Could you check a few things on this model? Use its own coordinates, in mm. Face numbers are marked on the shaded views. A direction names the side the tool comes from. Round coordinates to 2 decimals unless told otherwise and drop trailing zeros. Loops run counter-clockwise (first coordinate to the right, second up) from the corner with the lowest first, then second, coordinate; pieces in that order, holes last. Notation, with made-up numbers: (67.5, -12) - (84.5, -12) arc R21 cw to (84.5, -2) - close; hole circle Ø11 at (59, 28.25). An arc over 180 degrees is marked (long way). Use one line per item in the form item = value.
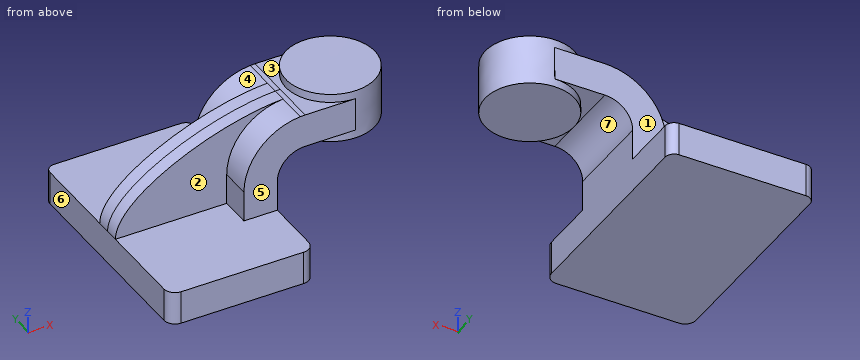
```python
from build123d import *

# Parameters (mm, degrees)
F1_DEPTH = 63.5
F2_DEPTH = 7.9375
F3_DEPTH = 25.4
F5_R     = 6.35
F6_R     = 5.08


with BuildPart() as f1:
    # F0 (on Front) → F1 (new body, symmetric)
    with BuildSketch(Plane.XZ):
        Polygon((-41.275, -9.525), (41.275, -9.525), (41.275, 9.525), (22.225, 9.525), (-41.275, 9.525), align=None)
    extrude(amount=F1_DEPTH, both=True)

    # F0 (on Front) → F2 (join, symmetric)
    with BuildSketch(Plane.XZ):
        with BuildLine():
            add(Edge.make_bspline(
                [(-41.275, 9.525), (-41.1638136776, 33.0921679971), (14.6157059848, 59.6638127103), (54.3682484127, 61.8142414647)],
                knots=[0, 0, 0, 0, 108.9382602659, 108.9382602659, 108.9382602659, 108.9382602659], degree=3))
            Line((-41.275, 9.525), (22.225, 9.525))
            Line((22.225, 9.525), (22.225, 27.0002))
            ThreePointArc((22.225, 27.0002), (31.489638553, 50.6920018607), (54.3682484127, 61.8142414647))
        make_face()
    extrude(amount=F2_DEPTH, both=True)

    # F0 (on Front) → F3 (join, symmetric)
    with BuildSketch(Plane.XZ):
        with BuildLine():
            Line((22.225, 9.525), (41.275, 9.525))
            Line((41.275, 9.525), (41.275, 27.0002))
            ThreePointArc((41.275, 27.0002), (45.9246798487, 38.2255201513), (57.15, 42.8752))
            Line((57.15, 42.8752), (60.325, 42.8752))
            Line((60.325, 42.8752), (60.325, 61.9252))
            Line((60.325, 61.9252), (57.15, 61.9252))
            add(Edge.make_bspline(
                [(54.3682484127, 61.8142414647), (55.3047053678, 61.8648994564), (56.2322683165, 61.902005145), (57.15, 61.9252)],
                knots=[108.9382602659, 108.9382602659, 108.9382602659, 108.9382602659, 111.5045361635, 111.5045361635, 111.5045361635, 111.5045361635], degree=3))
            ThreePointArc((54.3682484127, 61.8142414647), (31.489638553, 50.6920018607), (22.225, 27.0002))
            Line((22.225, 27.0002), (22.225, 9.525))
        make_face()
        Polygon((60.325, 61.9252), (60.325, 42.8752), (85.7332489532, 42.8752), (85.7661570114, 61.9252), align=None)
    extrude(amount=F3_DEPTH, both=True)

    # F0 (on Front) → F4 (revolve)
    with BuildSketch(Plane.XZ):
        Polygon((85.7661570114, 61.9252), (85.7332489532, 42.8752), (85.725, 38.1), (111.125, 38.1), (111.125, 66.675), (85.7743620872, 66.675), align=None)
    revolve(axis=Axis((85.7496810436, 0, 52.3875), (0.0017274545, 0, 0.9999985079)))

    # F5
    f5_edges = [f1.edges().sort_by_distance(p)[0] for p in [
        (41.275, -63.5, 0),
        (-41.275, -63.5, 0),
    ]]
    fillet(f5_edges, radius=F5_R)

    # F6
    f6_edges = [f1.edges().sort_by_distance(p)[0] for p in [
        (-41.275, 63.5, 0),
        (41.275, 63.5, 0),
    ]]
    fillet(f6_edges, radius=F6_R)


solid = f1.part
```
1. We'd pull the mould along X, two halves only. Please class the marked faces 5, 6 and 7: +X half, -X half, draft (parallel to the pull), parting line (faces both ways), or undercut.
Solution:
face_5 = draft
face_6 = -X half
face_7 = undercut
2. For P1, Ø5, axis at y = 32.5, z = 8.5, coming from the +X side (3 decimals); P2, Ø1.5, axis at x = 24, z = 33.5, coming from the +Y side; P3, Ø3, axis at y = 17.5, z = 43.5, coming from the +X side, each with a flat end and sliding along its axis, tell me the tip position at first contact or that it passes through.
Solution:
P1 = 41.275
P2 = 25.4
P3 = 105.45
3. On a 3-axis mill with a long thin cutter (end or side, diameter ignored), from which of +Z, -Z, +X, -X, +Y, -Y can I reach the whole of each face in a straight line? I mean the marked faces 1, 2, 3 and 4. Say none if no direction works.
Solution:
face_1 = +Z, +X, -X, +Y
face_2 = +Z, -X, -Y
face_3 = +Z, -X
face_4 = +Z, -X, +Y
4. If we section it at B-B, the plane y = -40: Write out the boundary of the cut face in (x, z) (3 decimals).
Solution:
outline = (-41.275, -9.525) - (41.275, -9.525) - (41.275, 9.525) - (-41.275, 9.525) - close
5. Please list where these lines run through material, in increasing order: line 1 along X through (y, z) = (-18, 4) (3 decimals); line 2 along Z through (x, y) = (2, 18) (3 decimals); line 3 along Y through (x, z) = (-15, 24).
Solution:
line_1 = -41.275 to 41.275
line_2 = -9.525 to 9.525
line_3 = -7.94 to 7.94
6. If we section it at A-A, the plane z = 1: Write out the boundary of the cut face in (x, y) (3 decimals), plus the area to 3 significant figures.
Solution:
outline = (-41.275, -57.15) arc R6.35 ccw to (-34.925, -63.5) - (34.925, -63.5) arc R6.35 ccw to (41.275, -57.15) - (41.275, 58.42) arc R5.08 ccw to (36.195, 63.5) - (-36.195, 63.5) arc R5.08 ccw to (-41.275, 58.42) - close
area = 10,500 mm^2
